Here's how the part is built. I have some questions about the finished solid (model axes, mm). Face numbers are marked on the shaded views. A direction names the side the tool comes from. Round coordinates to 2 decimals unless told otherwise and drop trailing zeros. Write each loop counter-clockwise with the first axis right and the second up, starting at its lowest first coordinate (ties: lowest second). Pieces come first, ordered by that corner, then holes. Notation, with made-up numbers: M 26.25,10.25 L 36.25,10.25 A32 ccw 36.25,48.25 Z; hole C 40,-1 d3. An arc over 180 degrees is marked long. Use one line per item in the form item = value. Start each with the question number.
Q1. I need wall thicknesses on line 1 along Y through (x, z) = (0.5, 28.5); line 2 along X through (y, z) = (-34, 38.5); line 3 along Y through (x, z) = (-4, -4). Which ranges of each line are inside material? Lowest first, please. Write a range as from..to.
Q2. For the marked faces 5, 6 and 7, which set-ups out of +Z, -Z, +X, -X, +Y, -Y let a thin tool reach every point of the face, with its end or its side?
Q3. I want a section at B-B on z = 20. State how many separate pieces and enclosed holes the cut face has, and give its area (3 significant figures).
Q4. I want a section at A-A on z = 102.5. List the corners of the cut face in (x, y) for me, and give its area (3 significant figures).
Q5. We'd pull the mould along X, two halves only. Please class the marked faces 1, 2, 3 and 4: +X half, -X half, draft (parallel to the pull), parting line (faces both ways), or undercut.
Q6. I'm going to push flat-ended pins straight in: pin 1 Ø12.5 at (y, z) = (-28, 21.5) entering from +X; pin 2 Ø6 at (x, z) = (16, -29) entering from -Y; pin 3 Ø1 at (y, z) = (-73.5, 32) entering from -X. Where does each tip first touch, or does it pass through?
```python
from build123d import *

# Parameters (mm, degrees)
F0_W      = 97.628775984
F0_H      = 23.3006943017
F3_DEPTH  = 118
F5_DEPTH  = 25
F6_W      = 12.4683696777
F6_H      = 23.7819701433
F7_DEPTH  = 25
F6_W_2    = 16.8170528486
F6_H_2    = 20.5661654472
F6_W_3    = 3.8202507421
F6_H_3    = 18.9904868603
F5_FACE_W = 12.4683696777
F5_FACE_H = 23.7819701433
F8_DEPTH  = 25
F9_W      = 15.9168411046
F9_H      = 16.453512013
F10_DEPTH = 25


with BuildPart() as f1:
    # F0 (on Top) → F1 (revolve)
    with BuildSketch(Plane.XY):
        with Locations((23.0226498097, 26.6735097393)):
            Rectangle(F0_W, F0_H)
    revolve(axis=Axis((24.7196350247, -32.6789328828, 0), (0.9918684705, -0.1272671882, 0)))

    # F2 (on Top) → F3 (join)
    with BuildSketch(Plane.XY):
        Polygon((0, -12.5550432131), (0, -59.4090670347), (40.5481569469, -58.6816631258), (40.5481569469, -16.4360441267), align=None)
    extrude(amount=F3_DEPTH)

    # F4 (on face) → F5 (join)
    with BuildSketch(Plane.XY.offset(118)):
        with BuildLine():
            ThreePointArc((38.9660080346, -51.5918619931), (37.4929859335, -44.804908652), (33.3389817945, -39.2392299533))
            ThreePointArc((33.3389817945, -39.2392299533), (23.254398026, -42.045514844), (13.6522556306, -37.8774306208))
            ThreePointArc((13.6522556306, -37.8774306208), (6.7419373602, -47.498950756), (8.1305858475, -59.2632103455))
            Line((8.1305858475, -59.2632103455), (37.3233440131, -58.7395138818))
            ThreePointArc((37.3233440131, -58.7395138818), (38.5500581705, -55.2588523329), (38.9660080346, -51.5918619931))
        make_face()
    extrude(amount=F5_DEPTH)

    # F6 (on face) → F7 (join)
    with BuildSketch(Plane(origin=(1.0654118014, -59.389954336, 0), x_dir=(0.9998391303, 0.0179363736, 0), z_dir=(0.0179363736, -0.9998391303, 0))):
        with Locations((26.5645338222, 119.3591877818)):
            Rectangle(F6_W, F6_H)
    extrude(amount=F7_DEPTH)

    # F6 (on face) + F5_face (on face) → F8 (join)
    with BuildSketch(Plane(origin=(1.0654118014, -59.389954336, 0), x_dir=(0.9998391303, 0.0179363736, 0), z_dir=(0.0179363736, -0.9998391303, 0))):
        with Locations((18.3676513843, 90.3412923217)):
            Rectangle(F6_W_2, F6_H_2)
        with Locations((26.5645338222, 119.3591877818)):
            Rectangle(F6_W, F6_H)
        with Locations((12.6832216047, 116.9634461403)):
            Rectangle(F6_W_3, F6_H_3)
    with BuildSketch(Plane(origin=(20.5226573435, -59.0409057594, 101.9755675833), x_dir=(0.9998391303, 0.0179363736, 0), z_dir=(0.0179363736, -0.9998391303, 0))):
        with BuildLine():
            add(Edge.make_bspline(
                [(-20.5259593482, -39.813077169), (-1.4657323401, -35.8130367899), (20.0287216176, -31.8741575877)],
                knots=[3.4641055883, 3.4641055883, 3.4641055883, 3.5071067631, 3.5071067631, 3.5071067631], degree=2, weights=[1, 0.9997688713, 1]))
            Line((20.0287216176, -31.8741575877), (20.0287216176, 16.0244324167))
            Line((20.0287216176, 16.0244324167), (16.8033898257, 16.0244324167))
            Line((16.8033898257, 16.0244324167), (16.8033898257, 41.0244324167))
            Line((16.8033898257, 41.0244324167), (-12.3940653254, 41.0244324167))
            Line((-12.3940653254, 41.0244324167), (-12.3940653254, 16.0244324167))
            Line((-12.3940653254, 16.0244324167), (-20.5259593482, 16.0244324167))
            Line((-20.5259593482, 16.0244324167), (-20.5259593482, -39.813077169))
        make_face()
        with Locations((7.1041576955, 17.3836201985)):
            Rectangle(F5_FACE_W, F5_FACE_H, mode=Mode.SUBTRACT)
    extrude(amount=F8_DEPTH)

    # F9 (on face) → F10 (join)
    with BuildSketch(Plane(origin=(-1.1907767819, -12.4410699495, 0), x_dir=(-0.9954507085, 0.095277946, 0), z_dir=(0.095277946, 0.9954507085, 0))):
        with Locations((-21.8754792586, 103.7665121257)):
            Rectangle(F9_W, F9_H)
    extrude(amount=F10_DEPTH)


solid = f1.part
```
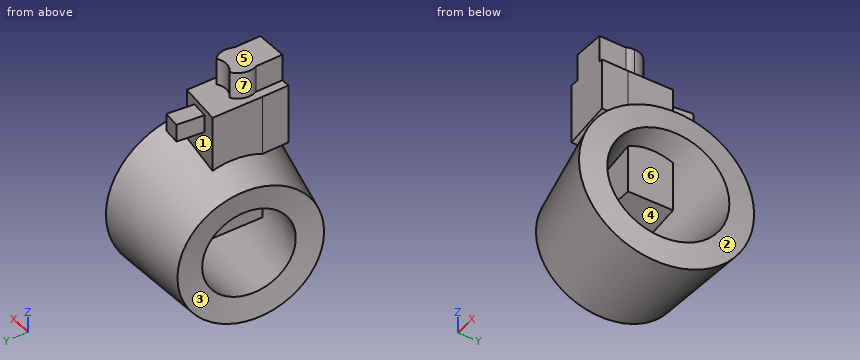
Reported:
q1.line_1 = -93.47..-65.39, -59.4..-12.6, 4.75..32.06
q1.line_2 = 0..40.55
q1.line_3 = -98.45..-74.3, 14.84..38.2
q2.face_5 = +Z, +X, -X, +Y, -Y
q2.face_6 = +X
q2.face_7 = +Z, -X
q3.separate_pieces = 3
q3.enclosed_holes = 0
q3.area = 6,670 mm^2
q4.outline = M 0,-59.41 L 0.45,-84.41 L 41,-83.68 L 40.55,-58.68 L 40.55,-16.44 L 28.51,-15.28 L 30.89,9.6 L 15.04,11.12 L 12.66,-13.77 L 0,-12.56 Z
q4.area = 3,220 mm^2
q5.face_1 = undercut
q5.face_2 = +X half
q5.face_3 = -X half
q5.face_4 = draft
q6.pin_1 = 40.55
q6.pin_2 = -99.02
q6.pin_3 = -39.52
